Work out the finished part from the listing and answer in its coordinate system (mm). A direction names the side the tool comes from. Round coordinates to 2 decimals unless told otherwise and drop trailing zeros. Order: outer loops, then holes, each group sorted by start corner. A loop starts at its lowest first (then second) coordinate and runs counter-clockwise, first axis right, second up. Notation, with made-up numbers: (-21, 52) -> (-11, 52) arc R30 ccw to (-11, 76) -> close; hole circle Ø9 at (-19.5, 14). An arc over 180 degrees is marked (long way). Use one line per item in the form item = value.
```python
from build123d import *

# Parameters (mm, degrees)
CUT_EXTRUDE_1_DEPTH = 3.3
FILLET_1_R          = 1
CHAMFER_1_SIZE      = 0.5


with BuildPart() as part:
    # 草图1 → 旋转1 (revolve)
    with BuildSketch(Plane.XY):
        Polygon((0, 0), (0, 6.5), (5.5, 6.5), (5.5, 4), (45.5, 4), (45.5, 3), (56.75, 3), (56.75, 0), align=None)
    revolve(axis=Axis((0, 0, 0), (1, 0, 0)))

    # 草图2 → 切除-拉伸1 (cut)
    with BuildSketch(Plane.ZY):
        Polygon((0, 2.309401077), (-2, 1.154700538), (-2, -1.154700538), (0, -2.309401077), (2, -1.154700538), (2, 1.154700538), align=None)
    extrude(amount=-CUT_EXTRUDE_1_DEPTH, mode=Mode.SUBTRACT)

    # 圆角1
    fillet_1_edges = [part.edges().sort_by_distance(p)[0] for p in [
        (0, -6.5, 0),
    ]]
    fillet(fillet_1_edges, radius=FILLET_1_R)

    # 倒角1
    chamfer_1_edges = [part.edges().sort_by_distance(p)[0] for p in [
        (56.75, -3, 0),
    ]]
    chamfer(chamfer_1_edges, length=CHAMFER_1_SIZE)


solid = part.part
```
Item 1: For faces 1 (the flat face through (1.63, -1.74, 0.99)), 2 (the flat face through (56.75, 0, 0)), 3 (the flat face through (5.5, 3, 3)), determine the directions among +Z, -Z, +X, -X, +Y, -Y from which every point of the face is accessible in a straight line to the end or side of a thin tool.
Findings:
face_1 = -X
face_2 = +Z, -Z, +X, +Y, -Y
face_3 = +X
Item 2: Consider line 1 along X through (y, z) = (2.5, 2.5); line 2 along X through (y, z) = (1, 1); line 3 along Y through (x, z) = (12, 0.75). Determine where each line is inside the solid, lowest interval first.
Findings:
line_1 = 0 to 45.5
line_2 = 3.3 to 56.75
line_3 = -3.93 to 3.93
Item 3: Flat-ended cylindrical pins translate along their axes: P1, Ø4, axis at x = 6.5, y = -0.5, coming from the +Z side; P2, Ø1.5, axis at x = 14.5, y = -4, coming from the +Z side; P3, Ø4, axis at x = 35.5, z = -0.5, coming from the -Y side; P4, Ø1.5, axis at x = 29, z = 1.5, coming from the -Y side. Find the tip coordinate at first contact, or state that the pin passes through.
Findings:
P1 = 6.5
P2 = 2.33
P3 = -4
P4 = -3.93
Item 4: Determine the mould class of faces 4 (the cylindrical face through (3.282, -5.158, -3.955)), 5 (the flat face through (3.3, 0, 0)), 6 (the flat face through (0, 0.1, -2.4)), 7 (the flat face through (2, 0, -2)) for opening direction Y: released by +Y, released by -Y, zero draft, split by the parting line, or undercut.
Findings:
face_4 = split by the parting line
face_5 = undercut
face_6 = zero draft
face_7 = undercut
Item 5: The part is cut by section C-C, the plane x = 31. Give the vertices of the cut face in (y, z).
Findings:
outline = circle Ø8 at (0, 0)
Item 6: The part is cut by section B-B, the plane x = 47.5. Give the vertices of the cut face in (y, z).
Findings:
outline = circle Ø6 at (0, 0)
Item 7: The part is cut by section A-A, the plane y = 0. Give the vertices of the cut face in (x, z), and give its area (3 significant figures).
Findings:
outline = (0, -5.5) arc R1 ccw to (1, -6.5) -> (5.5, -6.5) -> (5.5, -4) -> (45.5, -4) -> (45.5, -3) -> (56.25, -3) -> (56.75, -2.5) -> (56.75, 2.5) -> (56.25, 3) -> (45.5, 3) -> (45.5, 4) -> (5.5, 4) -> (5.5, 6.5) -> (1, 6.5) arc R1 ccw to (0, 5.5) -> (0, 2) -> (3.3, 2) -> (3.3, -2) -> (0, -2) -> close
area = 445 mm^2
